The listing builds one solid part. Answer for the finished solid, in the listing's coordinates (mm). A direction names the side the tool comes from. Round coordinates to 2 decimals unless told otherwise and drop trailing zeros. Write each loop counter-clockwise with the first axis right and the second up, starting at its lowest first coordinate (ties: lowest second). Pieces come first, ordered by that corner, then holes. Notation, with made-up numbers: M 74,-16.5 L 130,-16.5 A28 cw 130,1.5 Z; hole C 1,17 d5. An arc over 180 degrees is marked long. One line per item, written item: value. Start each with the question number.
(1) For a pull along Z with two mould halves and no side action, classify faces 1 (the flat face through (-6, 25.4, 0)), 2 (the flat face through (15, 6, 3.175)) as released by +Z, released by -Z, zero draft, split by the parting line, or undercut.
(2) Given P1, Ø4, axis at x = 11, y = 9, coming from the +Z side; P2, Ø2, axis at y = 8, z = -5, coming from the -X side; P3, Ø10, axis at x = 20, y = 5, coming from the -Z side; P4, Ø3, axis at y = 19, z = -1, coming from the +X side, each flat-ended and moving along its own axis, determine where each tip first touches the part or whether it passes through.
(3) Consider probe 1 along Y at (x, z) = (17, 0.5); probe 2 along Z at (x, y) = (-3, 17); probe 3 along Z at (x, y) = (5, 14.5). Determine where each line is inside the solid, lowest interval first.
(4) Section D-D (x = -19) is taken. Determine the outline of the cut face in (y, z).
(5) Section B-B (x = 11.5) is taken. Determine the outline of the cut face in (y, z) (3 decimals).
(6) Section A-A (y = 17) is taken. Determine the outline of the cut face in (x, z) (3 decimals).
(7) Section C-C (z = -15) is taken. Determine the outline of the cut face in (x, y), plus the area to 3 significant figures.
(8) For faces 3 (the flat face through (-6, 0, 0)), 4 (the flat face through (-5.499, 13, 0)), 5 (the flat face through (15, 12.7, 0)), determine the directions among +Z, -Z, +X, -X, +Y, -Y from which every point of the face is accessible in a straight line to the end or side of a thin tool.
```python
from build123d import *

# Parameters (mm, degrees)
BOSS_EXTRUDE1_DEPTH = 25.4
CUT_EXTRUDE1_DEPTH  = 12.7


with BuildPart() as part:
    # Sketch1 → Boss-Extrude1 (new body)
    with BuildSketch(Plane(origin=(0, 0, 0), x_dir=(1, 0, 0), z_dir=(0, 1, 0))):
        with BuildLine():
            Line((25.200781238, 3.175), (5.499261314, 3.175))
            Line((5.499261314, 3.175), (5.499261314, -3.175))
            Line((5.499261314, -3.175), (25.200781238, -3.175))
            ThreePointArc((25.200781238, -3.175), (25.350146385, -1.590621979), (25.4, 0))
            ThreePointArc((25.4, 0), (25.350146385, 1.590621979), (25.200781238, 3.175))
        make_face()
        with BuildLine():
            Line((0, 6.35), (5.499261314, 3.175))
            Line((5.499261314, 3.175), (25.200781238, 3.175))
            ThreePointArc((25.200781238, 3.175), (-25.4, 0), (25.200781238, -3.175))
            Line((25.200781238, -3.175), (5.499261314, -3.175))
            Line((5.499261314, -3.175), (0, -6.35))
            Line((0, -6.35), (-5.499261314, -3.175))
            Line((-5.499261314, -3.175), (-5.499261314, 3.175))
            Line((-5.499261314, 3.175), (0, 6.35))
        make_face()
    extrude(amount=BOSS_EXTRUDE1_DEPTH)

    # Sketch1_4 → Cut-Extrude1 (cut)
    with BuildSketch(Plane(origin=(0, 0, 0), x_dir=(1, 0, 0), z_dir=(0, 1, 0))):
        with BuildLine():
            Line((25.200781238, 3.175), (5.499261314, 3.175))
            Line((5.499261314, 3.175), (5.499261314, -3.175))
            Line((5.499261314, -3.175), (25.200781238, -3.175))
            ThreePointArc((25.200781238, -3.175), (25.350146385, -1.590621979), (25.4, 0))
            ThreePointArc((25.4, 0), (25.350146385, 1.590621979), (25.200781238, 3.175))
        make_face()
    extrude(amount=CUT_EXTRUDE1_DEPTH, mode=Mode.SUBTRACT)


solid = part.part
```
Recorded:
1. face 1: zero draft
1. face 2: undercut
2. P1: stops at z = 23.75
2. P2: stops at x = -25.08
2. P3: stops at z = -20.5
2. P4: stops at x = 25.4
3. probe 1: y = 12.7 to 25.4
3. probe 2: z = -25.22 to -4.62, 4.62 to 25.22
3. probe 3: z = -24.9 to -3.46, 3.46 to 24.9
4. outline: M 0,-16.86 L 25.4,-16.86 L 25.4,16.86 L 0,16.86 Z
5. outline: M 0,-22.648 L 25.4,-22.648 L 25.4,22.648 L 0,22.648 L 0,3.175 L 12.7,3.175 L 12.7,-3.175 L 0,-3.175 Z
6. outline: C 0,0 d50.8; hole M -5.499,-3.175 L 0,-6.35 L 5.499,-3.175 L 5.499,3.175 L 0,6.35 L -5.499,3.175 Z
7. outline: M -20.5,0 L 20.5,0 L 20.5,25.4 L -20.5,25.4 Z
7. area: 1,040 mm2
8. face 3: +Z, -Z, +X, -X, -Y
8. face 4: +Y, -Y
8. face 5: +X, -Y
